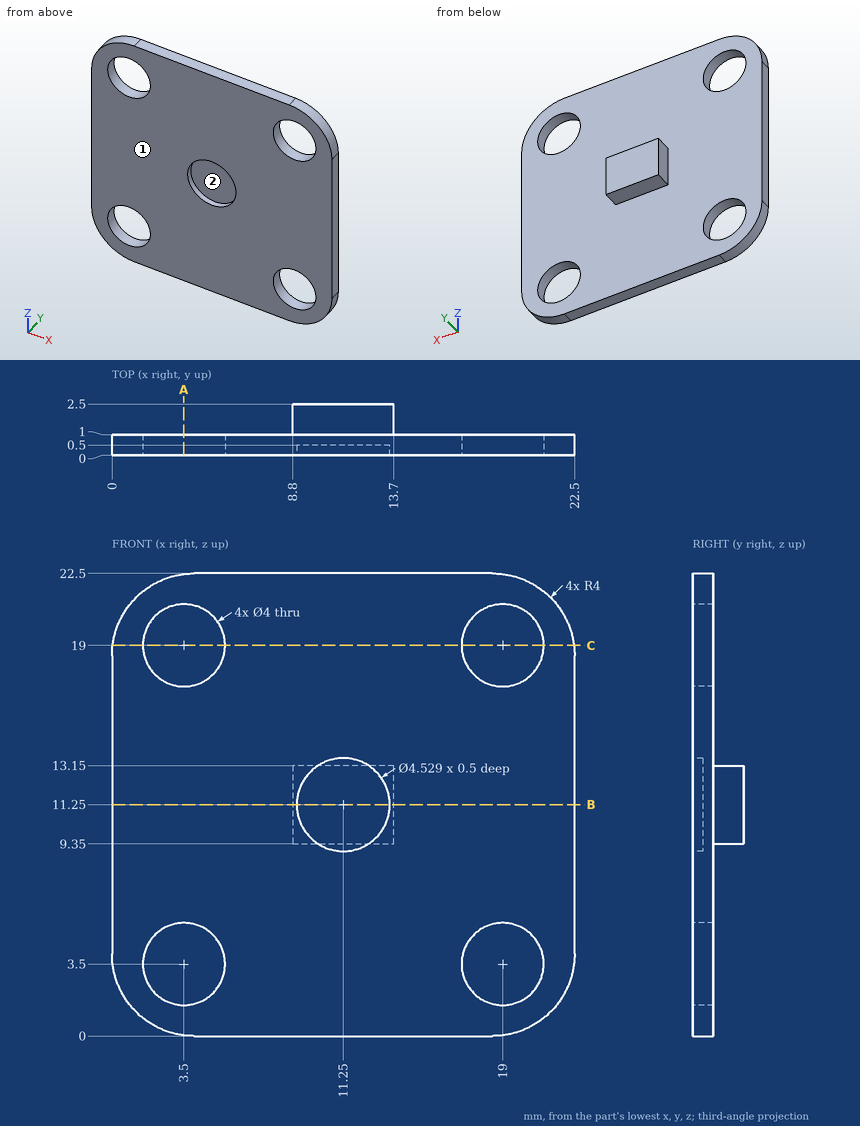
Print and shaded views of the part. All mm, measured from the part's lowest x, y and z. Coordinates: 2 decimals unless noted, no trailing zeros. Loops run counter-clockwise (first coordinate to the right, second up) from the corner with the lowest first, then second, coordinate; pieces in that order, holes last. Notation, with made-up numbers: (62.5, 23.25) - (69.5, 23.25) arc R26 ccw to (69.5, 39.25) - close; hole circle Ø3 at (87, 2.25). An arc over 180 degrees is marked (long way). Use one line per item in the form item = value. Start each with the question number.
1) Flat gauge pins, fed straight in: pin 1 (6.5 mm diameter, centred on x = 3.5, z = 3.5, fed in from +Y); pin 2 (0.8 mm diameter, centred on x = 11, y = 1.5, fed in from -Z); pin 3 (4 mm diameter, centred on x = 11.25, z = 11.25, fed in from -Y); pin 4 (7 mm diameter, centred on x = 15, z = 16, fed in from +Y). Where does each tip first touch, or does it go through?
2) Two-plate mould, pull along X, no slides. Class the marked faces 1 and 2: +X half, -X half, draft (parallel to the pull), parting line (faces both ways), or undercut.
3) Band-saw the part on B-B (z = 11.25). Give the cut face in (x, y) (1 decimal).
4) Band-saw the part on C-C (z = 19). Give the cut face in (x, y).
5) Band-saw the part on A-A (x = 3.5). Give the cut face in (y, z).
6) Drill centre lines: L1, parallel to X at y = 0.85, z = 3.5; L2, parallel to Z at x = 11.25, y = 0.3 (1 decimal). Where is each one in solid material? Low to high. Write a range as from..to.
Check values:
q1.pin_1 = 1
q1.pin_2 = 9.35
q1.pin_3 = 0.5
q1.pin_4 = 2.5
q2.face_1 = draft
q2.face_2 = undercut
q3.outline = (0, 0) - (9, 0) - (9, 0.5) - (13.5, 0.5) - (13.5, 0) - (22.5, 0) - (22.5, 1) - (13.7, 1) - (13.7, 2.5) - (8.8, 2.5) - (8.8, 1) - (0, 1) - close
q4.outline = (0.03, 0) - (1.5, 0) - (1.5, 1) - (0.03, 1) - close; (5.5, 0) - (17, 0) - (17, 1) - (5.5, 1) - close; (21, 0) - (22.47, 0) - (22.47, 1) - (21, 1) - close
q5.outline = (0, 0.03) - (1, 0.03) - (1, 1.5) - (0, 1.5) - close; (0, 5.5) - (1, 5.5) - (1, 17) - (0, 17) - close; (0, 21) - (1, 21) - (1, 22.47) - (0, 22.47) - close
q6.L1 = 0.03..1.5, 5.5..17, 21..22.47
q6.L2 = 0..9, 13.5..22.5
